The model under review builds one solid part; all positions refer to its coordinate system, in mm. A direction names the side the tool comes from. Coordinates: 2 decimals unless noted, no trailing zeros. Write each loop counter-clockwise with the first axis right and the second up, starting at its lowest first coordinate (ties: lowest second). Pieces come first, ordered by that corner, then holes. Notation, with made-up numbers: (67.5, 33.5) -> (96.5, 33.5) arc R11 cw to (96.5, 40.5) -> close; hole circle Ø8 at (-38, 4). An arc over 180 degrees is marked (long way). Write each question's results on one line, items separated by ' | '.
Autodesk Inventor part; units mm, degrees
ref_plane "YZ Plane" through (0, 0, 0) normal (1, 0, 0) x (0, 1, 0)
ref_plane "XZ Plane" through (0, 0, 0) normal (0, 1, 0) x (-1, 0, 0)
ref_plane "XY Plane" through (0, 0, 0) normal (0, 0, 1) x (1, 0, 0)
sketch "Sketch2" plane through (0, 0, 0) normal (0, 1, 0) x (-1, 0, 0)
  line L0 (-1.5, 6) -> (1.5, 6)
  line L1 (1.5, 6) -> (1.5, -6)
  line L2 (1.5, -6) -> (-1.5, -6)
  line L3 (-1.5, -6) -> (-1.5, 6)
  line L4 (-1.5, 6) -> (1.5, -6) construction
  line L5 (1.5, 6) -> (-1.5, -6) construction
  line L6 (1.5, 0) -> (-1.5, 0)
  circle A0 centre (-1, 3) radius 0.8
  circle A1 centre (-1, -3) radius 0.8
  line L7 (-4.5, -9) -> (4.5, -9)
  line L8 (4.5, -9) -> (4.5, 9)
  line L9 (4.5, 9) -> (-4.5, 9)
  line L10 (-4.5, 9) -> (-4.5, -9)
  line L11 (-4.5, -9) -> (4.5, 9) construction
  line L12 (4.5, -9) -> (-4.5, 9) construction
  point P0 (0, 0)
  dimension "d2" = 3
  dimension "d3" = 12
  dimension "d4" = 1.6
  dimension "d5" = 2.5
  dimension "d6" = 3
  dimension "d7" = 9
  dimension "d8" = 18
extrude "Extrusion2" add sketch "Sketch2" along normal blind 2 contours L0 L1 L6 L3 A0 | A0 L3 | L1 L2 L3 A1 L6 | A1 L3 picked at (-1.0814, 3.2162) picked at (-1.0814, -2.7838)
extrude "Extrusion3" add sketch "Sketch2" along normal blind 8 contours L3 A0 | L3 A1 | L10 L9 L8 L7 picked at (-1.5421, 2.834) picked at (-1.5421, -3.166)
fillet "Fillet1" radius 2 8 edges at (-4.5, 0, 0) (0, 0, -9) (4.5, 0, 0) (0, 0, 9) (-4.5, 4, -9) (-4.5, 4, 9) (4.5, 4, 9) (4.5, 4, -9)
sketch "Sketch4" plane through (-4.5, 0, -9) normal (-1, 0, 0) x (0, 0, 1)
  line L0 (0, 0) -> (18, 0) construction
  line L1 (18, 0) -> (18, 8) construction
  line L2 (0, 0) -> (18, 0) construction
  line L3 (18, 0) -> (18, 2) construction
  line L4 (18, 2) -> (0, 2) construction
  line L5 (0, 2) -> (0, 0) construction
  line L6 (9, 0) -> (9, 8)
  line L7 (0, 8) -> (18, 8) construction
  circle A0 centre (6, 4.5) radius 1
  circle A1 centre (12, 4.5) radius 1
  dimension "d13" = 2
  dimension "d15" = 2
  dimension "d16" = 6
  dimension "d17" = 2.5
extrude "Extrusion4" cut sketch "Sketch4" against normal through all
properties part number "Part1_3DPrint"
Q1. For line 1 (Y direction, x = -2.15, z = -3); line 2 (X direction, y = 6, z = -1.75); line 3 (Y direction, x = -0.5, z = 1.5), list the stretches that pass through material, from the lowest coordinate up. Write a range as from..to.
Solution:
line 1: 0..3.5, 5.5..8 | line 2: -4.5..-1.5, 1.5..4.5 | line 3: 0..2
Q2. Draft analysis for pull direction Y (two halves, no side actions). For faces 1 (the cylindrical face through (2.98, 5.49, -3.13)), 2 (the flat face through (-4.5, 5, 0)), 3 (the cylindrical face through (-3.93, 0.6, 0.1)), state which applies: pulls with the +Y half, pulls with the -Y half, needs draft (parallel to the pull), parting line crosses it, or undercut.
Solution:
face 1: undercut | face 2: needs draft | face 3: pulls with the -Y half
Q3. Add section A-A (y = 7). Write out the cut boundary in (x, z).
Solution:
outline: (-4.5, -7) arc R2 ccw to (-2.5, -9) -> (2.5, -9) arc R2 ccw to (4.5, -7) -> (4.5, 7) arc R2 ccw to (2.5, 9) -> (-2.5, 9) arc R2 ccw to (-4.5, 7) -> close; hole (-1.5, -6) -> (1.5, -6) -> (1.5, 6) -> (-1.5, 6) -> close
Q4. Add section B-B (z = 3). Write out the cut boundary in (x, y), plus the area to 3 significant figures.
Solution:
outline: (-4.5, 2) arc R2 ccw to (-2.5, 0) -> (2.5, 0) arc R2 ccw to (4.5, 2) -> (4.5, 3.5) -> (1.5, 3.5) -> (1.5, 2) -> (-1.5, 2) -> (-1.5, 3.5) -> (-4.5, 3.5) -> close; (-4.5, 5.5) -> (-1.5, 5.5) -> (-1.5, 8) -> (-4.5, 8) -> close; (1.5, 5.5) -> (4.5, 5.5) -> (4.5, 8) -> (1.5, 8) -> close | area: 40.3 mm²
Q5. Machinability: for faces 4 (the cylindrical face through (3.9, 5.04, 8.43)), 5 (the flat face through (0, 5, -6)), which of the approach directions +Z, -Z, +X, -X, +Y, -Y give a long, thin tool a straight path to every point of the face, cutting with its end or side? Answer none if there is none.
Solution:
face 4: +Z, +X, +Y, -Y | face 5: +Y
Q6. Clearance check with flat-ended pins moving along their axes: P1, Ø2.5, axis at y = 4.5, z = 3, coming from the -X side; P2, Ø1.8, axis at y = 4.5, z = -3, coming from the +X side; P3, Ø1.5, axis at x = -0.5, z = -0.5, coming from the +Y side. State where each tip first meets the part, or that it passes through.
Solution:
P1: x = -4.5 | P2: through | P3: y = 2
Q7. Add section C-C (x = 2). Write out the cut boundary in (y, z), plus the area to 3 significant figures.
Solution:
outline: (0, -7) arc R2 ccw to (2, -9) -> (8, -9) -> (8, 9) -> (2, 9) arc R2 ccw to (0, 7) -> close; hole circle Ø2 at (4.5, -3); hole circle Ø2 at (4.5, 3) | area: 136 mm²
Q8. Add section D-D (y = 4.5). Write out the cut boundary in (x, z).
Solution:
outline: (-4.5, -7) arc R2 ccw to (-2.5, -9) -> (2.5, -9) arc R2 ccw to (4.5, -7) -> (4.5, -4) -> (1.5, -4) -> (1.5, -6) -> (-1.5, -6) -> (-1.5, -4) -> (-4.5, -4) -> close; (-4.5, -2) -> (-1.5, -2) -> (-1.5, 2) -> (-4.5, 2) -> close; (-4.5, 4) -> (-1.5, 4) -> (-1.5, 6) -> (1.5, 6) -> (1.5, 4) -> (4.5, 4) -> (4.5, 7) arc R2 ccw to (2.5, 9) -> (-2.5, 9) arc R2 ccw to (-4.5, 7) -> close; (1.5, -2) -> (4.5, -2) -> (4.5, 2) -> (1.5, 2) -> close
